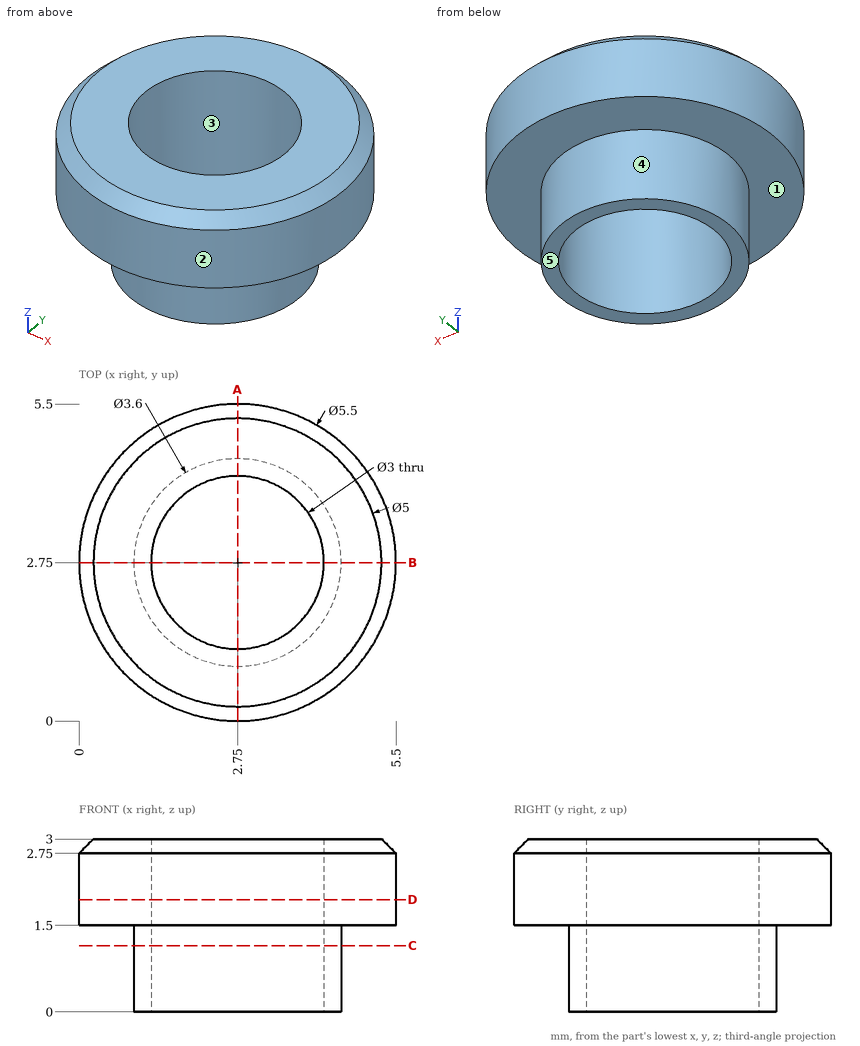
Check sheet for the drawn part. Datum: minimum x, y, z corner. Units: mm. A direction names the side the tool comes from. Round coordinates to 2 decimals unless told otherwise and drop trailing zeros. Loops run counter-clockwise (first coordinate to the right, second up) from the corner with the lowest first, then second, coordinate; pieces in that order, holes last.
Item 1: Cross-section at D-D on z = 1.95. Record the boundary of the cut face in (x, y), then the cut area to 3 significant figures.
Item 2: Gauge pin test, flat ends, axial feed: pin 1 (1 mm diameter, centred on x = 3, z = 0.5, fed in from +Y); pin 2 (1.5 mm diameter, centred on y = 4.5, z = 2.5, fed in from -X); pin 3 (1.5 mm diameter, centred on x = 1.5, y = 3.5, fed in from -Z). Record the tip position at first contact, or that the pin passes through.
Item 3: Mould release check, pull along Y, two halves, no side actions. Record for the marked faces 1, 2 and 3: pulls with the +Y half, pulls with the -Y half, needs draft (parallel to the pull), parting line crosses it, or undercut.
Item 4: Thickness scan on line 1 (Y direction, x = 2.75, z = 1); line 2 (Y direction, x = 2.75, z = 2.2). Record the ranges inside material, lowest first.
Item 5: Cross-section at A-A on x = 2.75. Record the boundary of the cut face in (y, z).
Item 6: Access from +Z, -Z, +X, -X, +Y, -Y to the whole of each face (thin tool, end or side, straight path). Record for the marked faces 4 and 5.
Item 7: Cross-section at C-C on z = 1.15. Record the boundary of the cut face in (x, y).
Answer sheet:
1. outline: circle Ø5.5 at (2.75, 2.75); hole circle Ø3 at (2.75, 2.75)
1. area: 16.7 mm2
2. pin 1: stops at y = 4.55
2. pin 2: stops at x = 0.19
2. pin 3: stops at z = 0
3. face 1: needs draft
3. face 2: parting line crosses it
3. face 3: undercut
4. line 1: y = 0.95 to 1.25, 4.25 to 4.55
4. line 2: y = 0 to 1.25, 4.25 to 5.5
5. outline: (0, 1.5) - (0.95, 1.5) - (0.95, 0) - (1.25, 0) - (1.25, 3) - (0.25, 3) - (0, 2.75) - close; (4.25, 0) - (4.55, 0) - (4.55, 1.5) - (5.5, 1.5) - (5.5, 2.75) - (5.25, 3) - (4.25, 3) - close
6. face 4: -Z
6. face 5: -Z, +X, -X, +Y, -Y
7. outline: circle Ø3.6 at (2.75, 2.75); hole circle Ø3 at (2.75, 2.75)
